Input: dimensioned drawing with shaded views. Units: mm. Origin: part minimum x, y, z. A direction names the side the tool comes from. Round coordinates to 2 decimals unless told otherwise and drop trailing zeros. Loops run counter-clockwise (first coordinate to the right, second up) from the corner with the lowest first, then second, coordinate; pieces in that order, holes last. Notation, with made-up numbers: M 76,23 L 102,23 A24 ccw 102,33 Z; hole C -24,53.25 d11. An arc over 180 degrees is marked long. Put each result on its own line as item: value. Start each with the question number.
1) Section A-A on z = 5. Output: boundary loops of the cut face in (x, y) (1 decimal).
2) Line query: probe 1 along Y at (x, z) = (21.25, 6.75); probe 2 along X at (y, z) = (11.25, 5.5) (1 decimal); probe 3 along Z at (x, y) = (20, 11.25). Output: solid intervals per line, ascending.
3) Reachability of the marked faces 1, 2 and 3 from +Z, -Z, +X, -X, +Y, -Y: full face, straight path, thin tool, end or side. Return the list, or none.
4) Section D-D on z = 9. Output: boundary loops of the cut face in (x, y) (1 decimal).
5) Pin query (flat end, axial travel): pin 1 (2 mm diameter, centred on x = 4, z = 1.5, fed in from +Y); pin 2 (2.5 mm diameter, centred on x = 22, z = 5.5, fed in from +Y); pin 3 (6 mm diameter, centred on x = 12.5, z = 1, fed in from +Y). Return the tip coordinate at first contact, or that it passes through.
6) Section C-C on y = 9.5. Output: boundary loops of the cut face in (x, z), plus the area to 3 significant figures.
7) Section B-B on x = 20. Output: boundary loops of the cut face in (y, z), plus the area to 3 significant figures.
8) Draft query along Y for the marked faces 4, 5, 6 and 7. Return one class per face: +Y half, -Y half, draft (parallel to the pull), parting line (faces both ways), or undercut.
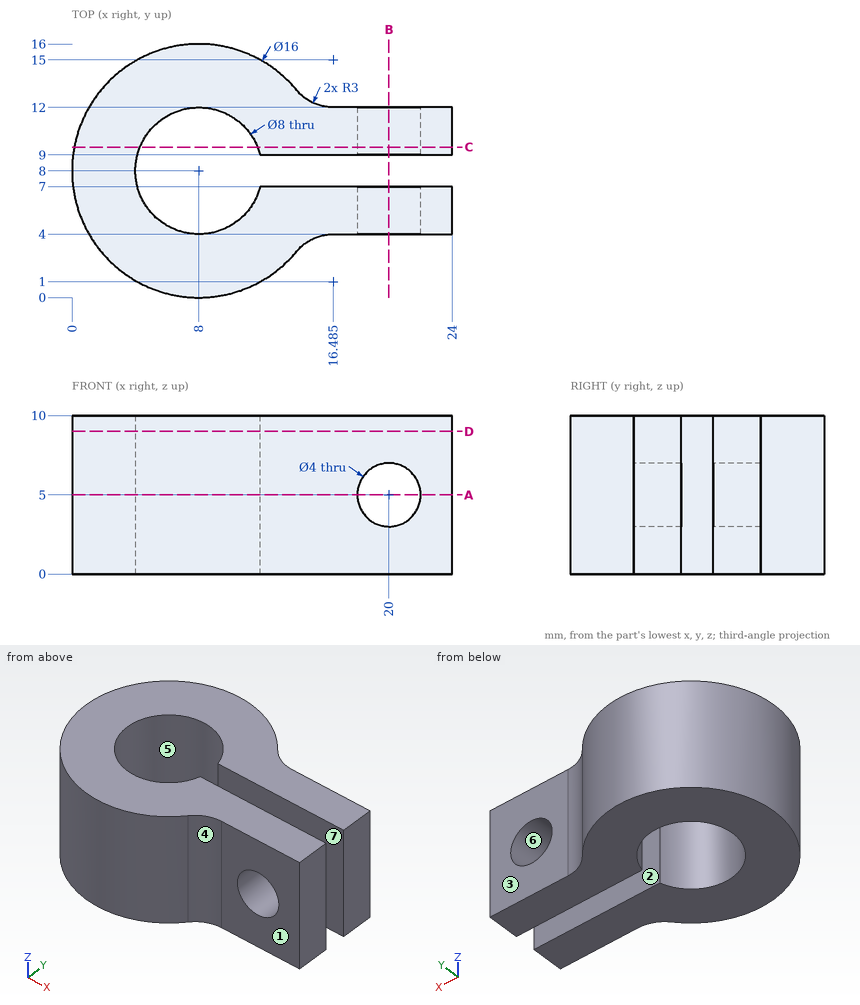
Geometry results:
1. outline: M 11.9,7 A4 cw long 11.9,9 L 18,9 L 18,12 L 16.5,12 A3 cw 14.2,13.1 A8 ccw long 14.2,2.9 A3 cw 16.5,4 L 18,4 L 18,7 Z; M 22,4 L 24,4 L 24,7 L 22,7 Z; M 22,9 L 24,9 L 24,12 L 22,12 Z
2. probe 1: y = 4 to 7, 9 to 12
2. probe 2: x = 0.7 to 5.7, 10.3 to 18.1, 21.9 to 24
2. probe 3: z = 0 to 3, 7 to 10
3. face 1: +Z, -Z, +X, -Y
3. face 2: +Z, -Z, +X
3. face 3: +Z, -Z, +X, +Y
4. outline: M 11.9,7 A4 cw long 11.9,9 L 24,9 L 24,12 L 16.5,12 A3 cw 14.2,13.1 A8 ccw long 14.2,2.9 A3 cw 16.5,4 L 24,4 L 24,7 Z
5. pin 1: stops at y = 15.42
5. pin 2: stops at y = 12
5. pin 3: stops at y = 15.86
6. outline: M 0.14,0 L 4.29,0 L 4.29,10 L 0.14,10 Z; M 11.71,0 L 24,0 L 24,10 L 11.71,10 Z; hole C 20,5 d4
6. area: 152 mm²
7. outline: M 4,0 L 7,0 L 7,3 L 4,3 Z; M 4,7 L 7,7 L 7,10 L 4,10 Z; M 9,0 L 12,0 L 12,3 L 9,3 Z; M 9,7 L 12,7 L 12,10 L 9,10 Z
7. area: 36.0 mm²
8. face 4: -Y half
8. face 5: undercut
8. face 6: draft
8. face 7: undercut
